For this review, take the finished solid that the model builds, in its own axes (mm). A direction names the side the tool comes from. Round coordinates to 2 decimals unless told otherwise and drop trailing zeros. Write each loop counter-clockwise with the first axis right and the second up, starting at its lowest first coordinate (ties: lowest second). Pieces come first, ordered by that corner, then holes.
from build123d import *

# Parameters (mm, degrees)
SKETCH1_R         = 456.61961
EXTRUDE1_DEPTH    = 106.59872
SKETCH2_R         = 279.38095
EXTRUDE2_DEPTH    = 7.46506
SKETCH3_R         = 327.70064
EXTRUDE3_DEPTH    = 234.73156
CHAMFER1_SIZE     = 69.85
CHAMFER1_SIZE2    = 51.89601
SKETCH4_R         = 223.63049
EXTRUDE4_DEPTH    = 333.86522
SKETCH5_R         = 435.62778
SKETCH5_R_2       = 377.02109
EXTRUDE5_DEPTH    = 1.34493
SKETCH6_R         = 29.36875
EXTRUDE6_DEPTH    = 105.71734
CIRPATTERN1_COUNT = 20
CHAMFER2_SIZE     = 6.35


with BuildPart() as part:
    # Sketch1 → Extrude1 (new body)
    with BuildSketch(Plane.XY):
        Circle(SKETCH1_R)
    extrude(amount=-EXTRUDE1_DEPTH)

    # Sketch2 → Extrude2 (cut)
    with BuildSketch(Plane.XY):
        Circle(SKETCH2_R)
    extrude(amount=-EXTRUDE2_DEPTH, mode=Mode.SUBTRACT)

    # Sketch3 → Extrude3 (add)
    with BuildSketch(Plane(origin=(0, 0, -106.59872), x_dir=(-1, 0, 0), z_dir=(0, 0, -1))):
        Circle(SKETCH3_R)
    extrude(amount=EXTRUDE3_DEPTH)

    # Chamfer1
    chamfer1_edges = [part.edges().sort_by_distance(p)[0] for p in [
        (327.70064, 0, -341.33028),
    ]]
    chamfer1_side = [part.faces().sort_by_distance(p)[0] for p in [
        (327.70064, 0, -223.9645),
    ]]
    chamfer(chamfer1_edges, length=CHAMFER1_SIZE, length2=CHAMFER1_SIZE2, reference=chamfer1_side[0])

    # Sketch4 → Extrude4 (cut)
    with BuildSketch(Plane.XY.offset(-7.46506)):
        Circle(SKETCH4_R)
    extrude(amount=-EXTRUDE4_DEPTH, mode=Mode.SUBTRACT)

    # Sketch5 → Extrude5 (cut)
    with BuildSketch(Plane.XY):
        Circle(SKETCH5_R)
        Circle(SKETCH5_R_2, mode=Mode.SUBTRACT)
    extrude(amount=-EXTRUDE5_DEPTH, mode=Mode.SUBTRACT)

    # Sketch6 → Extrude6 (cut)
    with BuildSketch(Plane.XY.offset(-1.34493)):
        with Locations((0, 406.44191)):
            Circle(SKETCH6_R)
    extrude6 = extrude(amount=-EXTRUDE6_DEPTH, mode=Mode.SUBTRACT)

    # CirPattern1: Extrude6 ×20 about axis
    cirpattern1_axis = Axis((0, 0, 0), (0, 0, 1))
    for i in range(1, CIRPATTERN1_COUNT):
        add(extrude6.rotate(cirpattern1_axis, i * 360 / CIRPATTERN1_COUNT), mode=Mode.SUBTRACT)

    # Chamfer2
    chamfer2_edges = [part.edges().sort_by_distance(p)[0] for p in [
        (-223.63049, 0, -341.33028),
    ]]
    chamfer(chamfer2_edges, length=CHAMFER2_SIZE)


solid = part.part
(1) For faces 1 (the face through (-208, 84, -7.465)), 2 (the face through (-130.96, -415.424, -53.235)), list the 3-axis set-ups (+Z, -Z, +X, -X, +Y, -Y) from which the entire face can be reached by the end or side of a thin tool; tool diameter is ignored.
Geometry check:
face 1: +Z
face 2: +Z, -Z
(2) For line 1 along Y through (x, z) = (0, -3.25); line 2 along X through (y, z) = (225, -56.5); line 3 along X through (y, z) = (-308.5, -101.5), list the stretches that pass through material, from the lowest coordinate up.
Geometry check:
line 1: y = -456.62 to -435.81, -377.07 to -279.38, 279.38 to 377.07, 435.81 to 456.62
line 2: x = -397.34 to -354.69, -302.95 to 302.95, 354.69 to 397.34
line 3: x = -336.64 to -260.11, -217.69 to 217.69, 260.11 to 336.64
(3) Mouldability with a two-part tool opening along X and no side actions: class faces 3 (the face through (-259.11, 350.13, -53.24)), 4 (the face through (-3.82, 435.56, -53.24)), 5 (the face through (404, -167, 0)), 6 (the face through (210.7, -405.1, -52.6)) as pulls with the +X half, pulls with the -X half, needs draft (parallel to the pull), parting line crosses it, or undercut.
Geometry check:
face 3: undercut
face 4: undercut
face 5: needs draft
face 6: parting line crosses it
(4) For pin 1 Ø3 at (x, z) = (219, -64) entering from +Y; pin 2 Ø1.7 at (x, y) = (414.5, 135.5) entering from -Z; pin 3 Ø8 at (x, z) = (-125, -97) entering from -Y, all flat-tipped, find the tip position at first contact; note any pin that passes through.
Geometry check:
pin 1: stops at y = 401.49
pin 2: stops at z = -106.6
pin 3: stops at y = -440.3
(5) We need section A-A, the plane z = -231. Give the boundary of the cut face in (x, y).
Geometry check:
outline: circle Ø655.4 at (0, 0); hole circle Ø447.26 at (0, 0)
